```python
from build123d import *

# Parameters (mm, degrees)
SKETCH1_R           = 100
SKETCH1_R_2         = 6.9
SKETCH1_R_3         = 10.75
SKETCH1_R_4         = 3
SKETCH1_R_5         = 2.25
SKETCH1_R_6         = 7
BOSS_EXTRUDE1_DEPTH = 6
SKETCH1_3_R         = 110
SKETCH1_3_R_2       = 100
BOSS_EXTRUDE2_DEPTH = 100
FILLET1_R           = 10
SKETCH1_11_R        = 100
SKETCH1_11_R_2      = 6.9
SKETCH1_11_R_3      = 7
SKETCH1_11_R_4      = 2.25
SKETCH1_11_R_5      = 6.7
SKETCH1_11_R_6      = 14
BOSS_EXTRUDE7_DEPTH = 14
SKETCH7_R           = 30
CUT_EXTRUDE3_DEPTH  = 110


with BuildPart() as part:
    # Sketch1 → Boss-Extrude1 (new body)
    with BuildSketch(Plane.XY):
        Circle(SKETCH1_R)
        with Locations((30.882391056, 73.798901907)):
            Circle(SKETCH1_R_2, mode=Mode.SUBTRACT)
        with Locations((0, 80)):
            Circle(SKETCH1_R_3, mode=Mode.SUBTRACT)
        with Locations((-31.073387423, 73.718685515)):
            Circle(SKETCH1_R_4, mode=Mode.SUBTRACT)
        with Locations((-49.00574775, 63.233192925)):
            Circle(SKETCH1_R_5, mode=Mode.SUBTRACT)
        with Locations((51.329760909, 61.361678962)):
            Circle(SKETCH1_R_6, mode=Mode.SUBTRACT)
    extrude(amount=BOSS_EXTRUDE1_DEPTH)

    # Sketch1<3> → Boss-Extrude2 (add)
    with BuildSketch(Plane.XY):
        Circle(SKETCH1_3_R)
        Circle(SKETCH1_3_R_2, mode=Mode.SUBTRACT)
    extrude(amount=BOSS_EXTRUDE2_DEPTH)

    # Fillet1
    fillet1_edges = [part.edges().sort_by_distance(p)[0] for p in [
        (-110, 0, 0),
    ]]
    fillet(fillet1_edges, radius=FILLET1_R)

    # Sketch1<11> → Boss-Extrude7 (add)
    with BuildSketch(Plane.XY):
        Circle(SKETCH1_11_R)
        with Locations((30.882391056, 73.798901907)):
            Circle(SKETCH1_11_R_2, mode=Mode.SUBTRACT)
        with Locations((51.329760909, 61.361678962)):
            Circle(SKETCH1_11_R_3, mode=Mode.SUBTRACT)
        with Locations((-49.00574775, 63.233192925)):
            Circle(SKETCH1_11_R_4, mode=Mode.SUBTRACT)
        with Locations((-31.073387423, 73.718685515)):
            Circle(SKETCH1_11_R_5, mode=Mode.SUBTRACT)
        with Locations((0, 80)):
            Circle(SKETCH1_11_R_6, mode=Mode.SUBTRACT)
    extrude(amount=BOSS_EXTRUDE7_DEPTH)

    # Sketch7 → Cut-Extrude3 (cut)
    with BuildSketch(Plane.XY.offset(14)):
        Circle(SKETCH7_R)
    extrude(amount=-CUT_EXTRUDE3_DEPTH, mode=Mode.SUBTRACT)


solid = part.part
```
Read the model definition and answer for the solid it produces. Units are mm, in the model's axes. A direction names the side the tool comes from. Give positions to 0.01 mm unless a question says otherwise; leave off trailing zeros. Write each loop counter-clockwise with the first axis right and the second up, starting at its lowest first coordinate (ties: lowest second). Pieces come first, ordered by that corner, then holes. Notation, with made-up numbers: M -27.75,5.5 L 7.25,5.5 A16 ccw 7.25,26.5 Z; hole C 24,88.25 d2. An arc over 180 degrees is marked long. Put each result on its own line as item: value. Start each with the question number.
1. The part is cut by section B-B, the plane x = 0. Give the vertices of the cut face in (y, z).
2. The part is cut by section C-C, the plane z = 77.5. Give the vertices of the cut face in (x, y), and give its area (3 significant figures).
3. Consider line 1 along Y through (x, z) = (0, 11); line 2 along Y through (x, z) = (0, 1); line 3 along Y through (x, z) = (-1, 69.5) (3 decimals). Determine where each line is inside the solid, lowest interval first.
4. For a pull along Y with two mould halves and no side action, classify faces 3 (the flat face through (23.9, -97.3, 100)), 4 (the cylindrical face through (-23.846, -107.384, 54.37)), 5 (the cylindrical face through (95.38, 30.04, 56.4)) as released by +Y, released by -Y, zero draft, split by the parting line, or undercut.
5. The part is cut by section A-A, the plane y = 0. Give the vertices of the cut face in (x, z), and give its area (3 significant figures).
6. Each of these flat-tipped pins is pushed along its axis until it touches: pin 1 Ø8 at (x, z) = (-49.5, 36.5) entering from +Y; pin 2 Ø2 at (y, z) = (45, 62.5) entering from -X; pin 3 Ø6 at (x, y) = (47.5, -43.5) entering from +Z. Where does it stop, or does it pass through?
7. Which of the six approach directions +Z, -Z, +X, -X, +Y, -Y give full straight-line access (tool end or side, diameter ignored) to faces 1 (the flat face through (4.1, 69.7, 6)), 2 (the cylindrical face through (55.093, 67.264, 6.902))?
Final values:
1. outline: M -110,10 A10 ccw -100,0 L -30,0 L -30,14 L -100,14 L -100,100 L -110,100 Z; M 30,0 L 69.25,0 L 69.25,6 L 66,6 L 66,14 L 30,14 Z; M 90.75,0 L 100,0 A10 ccw 110,10 L 110,100 L 100,100 L 100,14 L 94,14 L 94,6 L 90.75,6 Z
2. outline: C 0,0 d220; hole C 0,0 d200
2. area: 6,600 mm²
3. line 1: y = -110 to -30, 30 to 66, 94 to 110
3. line 2: y = -104.36 to -30, 30 to 69.25, 90.75 to 104.36
3. line 3: y = -109.995 to -99.995, 99.995 to 109.995
4. face 3: zero draft
4. face 4: split by the parting line
4. face 5: undercut
5. outline: M -110,10 A10 ccw -100,0 L -30,0 L -30,14 L -100,14 L -100,100 L -110,100 Z; M 30,0 L 100,0 A10 ccw 110,10 L 110,100 L 100,100 L 100,14 L 30,14 Z
5. area: 3,920 mm²
6. pin 1: stops at y = 100.15
6. pin 2: stops at x = -100.82
6. pin 3: stops at z = 14
7. face 1: +Z
7. face 2: +Z, -Z
